Autodesk Inventor part; units mm, degrees
ref_plane "YZ Plane" through (0, 0, 0) normal (1, 0, 0) x (0, 1, 0)
ref_plane "XZ Plane" through (0, 0, 0) normal (0, 1, 0) x (-1, 0, 0)
ref_plane "XY Plane" through (0, 0, 0) normal (0, 0, 1) x (1, 0, 0)
sketch "Skizze1" plane through (0, 0, 0) normal (1, 0, 0) x (0, 1, 0)
  line L0 (25, 70) -> (-25, 70)
  line L1 (-25, 70) -> (-25, -70)
  line L2 (-25, -70) -> (25, -70)
  line L3 (25, -70) -> (25, 70)
  line L4 (25, 70) -> (-25, -70) construction
  line L5 (-25, 70) -> (25, -70) construction
  point P0 (0, 0)
  dimension "d0" = 140
  dimension "d1" = 50
extrude "Extrusion1" add sketch "Skizze1" along normal blind 2
sketch "Skizze2" plane through (2, 0, 0) normal (1, 0, 0) x (0, 0, -1)
  circle A0 centre (-60.5, 20) radius 2.5
  circle A1 centre (-60.5, -20) radius 2.5
  circle A2 centre (60.5, 20) radius 2.5
  circle A3 centre (60.5, -20) radius 2.5
  point P0 (0, 0)
  dimension "d4" = 5
  dimension "d5" = 5
  dimension "d6" = 5
  dimension "d7" = 5
  dimension "d8" = 121
  dimension "d9" = 60.5
  dimension "d10" = 121
  dimension "d11" = 60.5
  dimension "d12" = 40
  dimension "d13" = 20
extrude "Extrusion2" cut sketch "Skizze2" against normal blind 2
sketch "Skizze3" plane through (2, 0, 0) normal (1, 0, 0) x (0, 0, -1)
  circle A0 centre (0, 0) radius 6.75
  circle A1 centre (9.5, 0) radius 1.25
  circle A2 centre (-9.5, 0) radius 1.25
  dimension "d16" = 2.5
  dimension "d17" = 2.5
  dimension "d18" = 13.5
  dimension "d19" = 19
  dimension "d20" = 9.5
extrude "Extrusion3" cut sketch "Skizze3" against normal blind 2
equation "\"d10\" = d8"
properties part number "Motorhalterplatte"
Can you work these out from the model? Positions are in its coordinate system, mm. Coordinates: 2 decimals unless noted, no trailing zeros. Write each loop counter-clockwise with the first axis right and the second up, starting at its lowest first coordinate (ties: lowest second). Pieces come first, ordered by that corner, then holes. Notation, with made-up numbers: M -3,85.5 L 27,85.5 A24 cw 27,119.5 Z; hole C -26,6 d10. An arc over 180 degrees is marked long. Write item = value, one per line. Start each with the question number.
Q1. If we section it at D-D, the plane y = 0: Write out the boundary of the cut face in (x, z), then the cut area to 3 significant figures.
Q2. Thinking about a two-plate mould opening in Y: for faces 1 (the face through (1.01, 0.05, 10.75)), 2 (the face through (2, -11, 1)), which applies, released by +Y, released by -Y, zero draft, split by the parting line, or undercut?
Q3. If we section it at C-C, the plane x = 1.6: Write out the boundary of the cut face in (y, z), then the cut area to 3 significant figures.
Q4. If we section it at A-A, the plane z = 9.5: Write out the boundary of the cut face in (x, y).
Q5. If I drill on L1, parallel to Y at x = 1.1, z = -60.5; L2, parallel to Y at x = 1.05, z = 0; L3, parallel to Y at x = 1.3, z = -9.5, over which ranges is the centre line in solid material (lowest first)? Write a range as [from, to].
Q6. If we section it at B-B, the plane y = 20: Write out the boundary of the cut face in (x, z).
Check sheet entries:
q1.outline = M 0,-70 L 2,-70 L 2,-10.75 L 0,-10.75 Z; M 0,-8.25 L 2,-8.25 L 2,-6.75 L 0,-6.75 Z; M 0,6.75 L 2,6.75 L 2,8.25 L 0,8.25 Z; M 0,10.75 L 2,10.75 L 2,70 L 0,70 Z
q1.area = 243 mm²
q2.face_1 = undercut
q2.face_2 = zero draft
q3.outline = M -25,-70 L 25,-70 L 25,70 L -25,70 Z; hole C -20,-60.5 d5; hole C -20,60.5 d5; hole C 0,0 d13.5; hole C 0,-9.5 d2.5; hole C 0,9.5 d2.5; hole C 20,-60.5 d5; hole C 20,60.5 d5
q3.area = 6,770 mm²
q4.outline = M 0,-25 L 2,-25 L 2,-1.25 L 0,-1.25 Z; M 0,1.25 L 2,1.25 L 2,25 L 0,25 Z
q5.L1 = [-25, -22.5], [-17.5, 17.5], [22.5, 25]
q5.L2 = [-25, -6.75], [6.75, 25]
q5.L3 = [-25, -1.25], [1.25, 25]
q6.outline = M 0,-70 L 2,-70 L 2,-63 L 0,-63 Z; M 0,-58 L 2,-58 L 2,58 L 0,58 Z; M 0,63 L 2,63 L 2,70 L 0,70 Z
